Build history of the part. All positions in model axes, mm. Face numbers are marked on the shaded views. A direction names the side the tool comes from. Round coordinates to 2 decimals unless told otherwise and drop trailing zeros. Write each loop counter-clockwise with the first axis right and the second up, starting at its lowest first coordinate (ties: lowest second). Pieces come first, ordered by that corner, then holes. Notation, with made-up numbers: (59.25, 75) -> (64.25, 75) arc R37 ccw to (64.25, 112) -> close; hole circle Ø2 at (-6.75, 33.5). An arc over 180 degrees is marked (long way). Answer in a Markdown table with one row per item.
```python
from build123d import *

# Parameters (mm, degrees)
BOSS_EXTRUDE1_DEPTH = 3


with BuildPart() as part:
    # Sketch1 → Boss-Extrude1 (new body)
    with BuildSketch(Plane.XY):
        with BuildLine():
            Line((-4.3, -163.694308418), (-4.3, -173.684305639))
            Line((-4.3, -173.684305639), (0.3, -173.684305639))
            Line((0.3, -173.684305639), (0.3, -163.694308418))
            Line((0.3, -163.694308418), (1.767652512, -163.694308418))
            ThreePointArc((1.767652512, -163.694308418), (3.479450891, -164.372291319), (4.262793246, -166.038511371))
            ThreePointArc((4.262793246, -166.038511371), (5.64620009, -171.458376258), (8.919091092, -175.994556853))
            ThreePointArc((8.919091092, -175.994556853), (9.496489466, -176.821698794), (9.7, -177.809694813))
            Line((9.7, -177.809694813), (9.7, -181.684305639))
            Line((9.7, -181.684305639), (-0.3, -181.684305639))
            Line((-0.3, -181.684305639), (-3.7, -181.684305639))
            Line((-3.7, -181.684305639), (-13.7, -181.684305639))
            Line((-13.7, -181.684305639), (-13.7, -177.809694813))
            ThreePointArc((-13.7, -177.809694813), (-13.496489466, -176.821698794), (-12.919091092, -175.994556853))
            ThreePointArc((-12.919091092, -175.994556853), (-9.64620009, -171.458376258), (-8.262793246, -166.038511371))
            ThreePointArc((-8.262793246, -166.038511371), (-7.479450891, -164.372291319), (-5.767652512, -163.694308418))
            Line((-5.767652512, -163.694308418), (-4.3, -163.694308418))
        make_face()
    extrude(amount=BOSS_EXTRUDE1_DEPTH)


solid = part.part
```
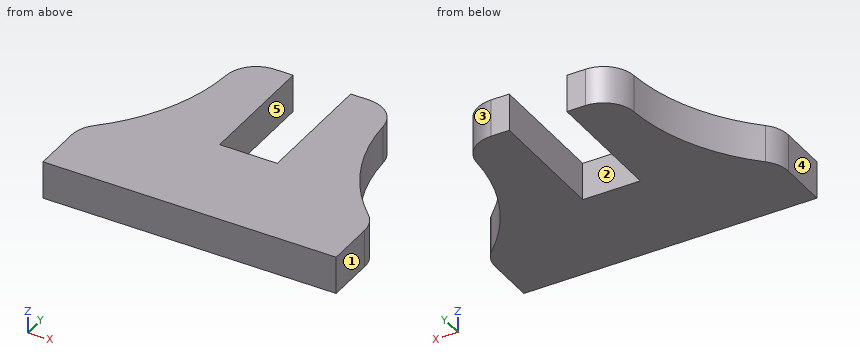
Q1. Two-plate mould, pull along X, no slides. Class the marked faces 3, 4 and 5: released by +X, released by -X, zero draft, split by the parting line, or undercut.
A:
| item | result |
|---|---|
| face 3 | released by +X |
| face 4 | released by -X |
| face 5 | undercut |
Q2. Drop flat-ended pins along their axis: P1, Ø1, axis at y = -175, z = 2, coming from the -X side; P2, Ø0.9, axis at x = -3, z = 1.5, coming from the +Y side. Give the stop position or say it passes through.
A:
| item | result |
|---|---|
| P1 | x = -12.42 |
| P2 | y = -173.68 |
Q3. Saw through at A-A on y = -169. Write the cut outline in (x, z).
A:
| item | result |
|---|---|
| outline | (-8.75, 0) -> (-4.3, 0) -> (-4.3, 3) -> (-8.75, 3) -> close; (0.3, 0) -> (4.75, 0) -> (4.75, 3) -> (0.3, 3) -> close |
Q4. Saw through at B-B on z = 0.25. Write the cut outline in (x, y), plus the area to 3 significant figures.
A:
| item | result |
|---|---|
| outline | (-13.7, -181.68) -> (9.7, -181.68) -> (9.7, -177.81) arc R2.5 ccw to (8.92, -175.99) arc R15 cw to (4.26, -166.04) arc R2.5 ccw to (1.77, -163.69) -> (0.3, -163.69) -> (0.3, -173.68) -> (-4.3, -173.68) -> (-4.3, -163.69) -> (-5.77, -163.69) arc R2.5 ccw to (-8.26, -166.04) arc R15 cw to (-12.92, -175.99) arc R2.5 ccw to (-13.7, -177.81) -> close |
| area | 269 mm² |
Q5. Saw through at D-D on y = -171.75. Write the cut outline in (x, z), plus the area to 3 significant figures.
A:
| item | result |
|---|---|
| outline | (-9.79, 0) -> (-4.3, 0) -> (-4.3, 3) -> (-9.79, 3) -> close; (0.3, 0) -> (5.79, 0) -> (5.79, 3) -> (0.3, 3) -> close |
| area | 32.9 mm² |
Q6. Saw through at C-C on x = -1.5. Write the cut outline in (y, z).
A:
| item | result |
|---|---|
| outline | (-181.68, 0) -> (-173.68, 0) -> (-173.68, 3) -> (-181.68, 3) -> close |
Q7. Which spindle directions (+Z, -Z, +X, -X, +Y, -Y) get a long thin tool onto all of the face, cutting with end or side? Do the marked faces 1 and 2. Say none if no direction does.
A:
| item | result |
|---|---|
| face 1 | +Z, -Z, +X, +Y, -Y |
| face 2 | +Z, -Z, +Y |
Q8. Wall check: line 1 (X direction, y = -172.5, z = 1.25); line 2 (X direction, y = -173.5, z = 1.7); line 3 (Y direction, x = 7.75, z = 1.3). Give the ranges that are in metal, low to high. Write a range as [from, to].
A:
| item | result |
|---|---|
| line 1 | [-10.18, -4.3], [0.3, 6.18] |
| line 2 | [-10.8, -4.3], [0.3, 6.8] |
| line 3 | [-181.68, -174.75] |
